Geometry check sheet. Reference: drawing and pictorial views, mm from the part's lowest x, y, z. A direction names the side the tool comes from. Coordinates: 2 decimals unless noted, no trailing zeros. Write each loop counter-clockwise with the first axis right and the second up, starting at its lowest first coordinate (ties: lowest second). Pieces come first, ordered by that corner, then holes. Notation, with made-up numbers: (2, 54) - (21, 54) arc R34 ccw to (21, 90) - close; hole circle Ø5 at (81, 88). An arc over 180 degrees is marked (long way). Use one line per item in the form item = value. Start each with the question number.
(1) Material ranges on line 1 (X direction, y = 17, z = 7.75) (1 decimal); line 2 (Y direction, x = 6.5, z = 6.5) (1 decimal); line 3 (X direction, y = 10.5, z = 3.5), recorded low to high. Write a range as [from, to].
(2) Sectioned sample at D-D (z = 5.5). Count the separate pieces of the cut face and the enclosed holes in it, and give its area (3 significant figures).
(3) Tool access check on the marked faces 1 and 2. Record the directions out of +Z, -Z, +X, -X, +Y, -Y that give a thin tool (end or side, any length) a straight path to the whole face; none if there is none.
(4) Mould release check, pull along X, two halves, no side actions. Record for the marked faces 3, 4 and 5: released by +X, released by -X, zero draft, split by the parting line, or undercut.
(5) Gauge pin test, flat ends, axial feed: pin 1 Ø1.5 at (x, y) = (16, 8.5) entering from -Z; pin 2 Ø2.5 at (x, y) = (16.73, 15.95) entering from +Z; pin 3 Ø2 at (x, z) = (18, 4.5) entering from -Y; pin 4 Ø4 at (x, z) = (14, 3) entering from +Y. Record the tip position at first contact, or that the pin passes through.
(6) Sectioned sample at A-A (x = 6). Record the cut outline in (y, z).
(7) Sectioned sample at B-B (y = 5.5). Record the cut outline in (x, z).
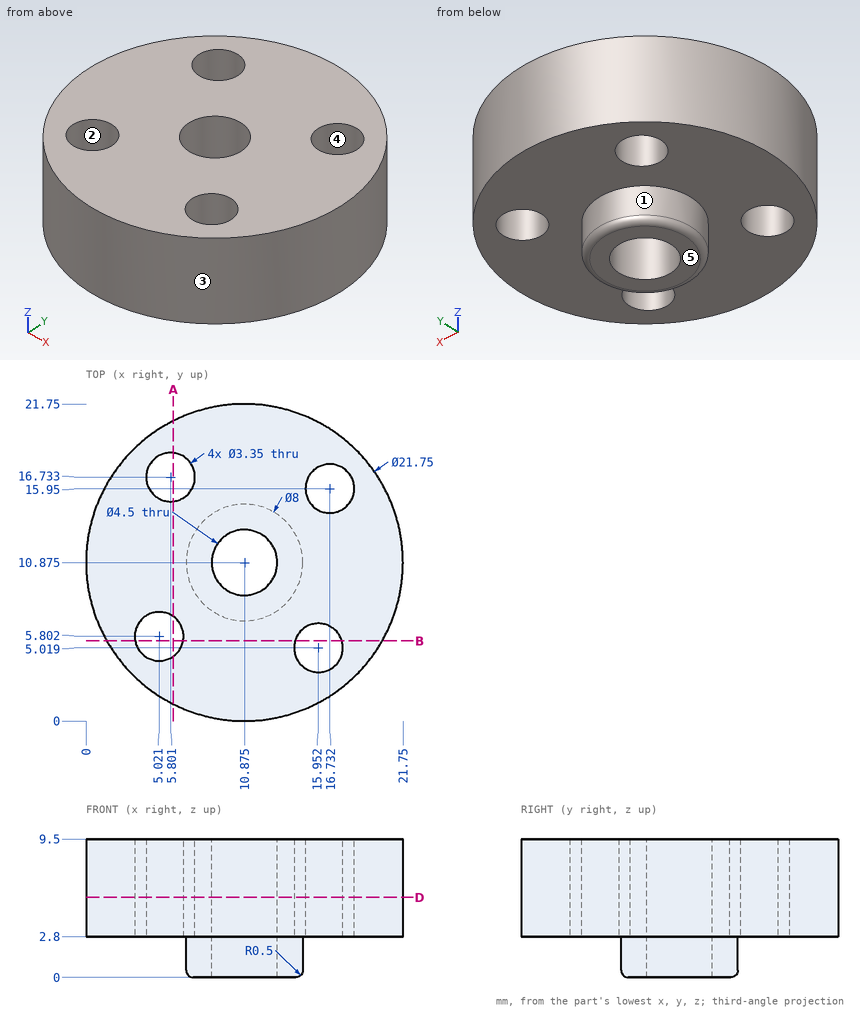
Answers below:
q1.line_1 = [1.9, 4.1], [7.5, 15.4], [18, 19.9]
q1.line_2 = [0.9, 5], [6.6, 15.2], [18.3, 20.8]
q1.line_3 = [0.01, 8.66], [13.09, 21.74]
q2.separate_pieces = 1
q2.enclosed_holes = 5
q2.area = 320 mm2
q3.face_1 = -Z
q3.face_2 = +Z, -Z
q4.face_3 = split by the parting line
q4.face_4 = undercut
q4.face_5 = zero draft
q5.pin_1 = 2.8
q5.pin_2 = through
q5.pin_3 = 1.89
q5.pin_4 = 21.69
q6.outline = (1.15, 2.8) - (4.44, 2.8) - (4.44, 9.5) - (1.15, 9.5) - close; (7.16, 2.8) - (15.07, 2.8) - (15.07, 9.5) - (7.16, 9.5) - close; (18.4, 2.8) - (20.6, 2.8) - (20.6, 9.5) - (18.4, 9.5) - close
q7.outline = (1.42, 2.8) - (3.37, 2.8) - (3.37, 9.5) - (1.42, 9.5) - close; (6.67, 2.8) - (14.35, 2.8) - (14.35, 9.5) - (6.67, 9.5) - close; (17.56, 2.8) - (20.33, 2.8) - (20.33, 9.5) - (17.56, 9.5) - close
